Part model, mm, in its own coordinate system. Give positions to 0.01 mm unless a question says otherwise; leave off trailing zeros. Order: outer loops, then holes, each group sorted by start corner. A loop starts at its lowest first (then second) coordinate and runs counter-clockwise, first axis right, second up. Notation, with made-up numbers: M 37.5,36 L 53.5,36 A12 ccw 53.5,53 Z; hole C 16.25,77 d11. An arc over 180 degrees is marked long. Answer as a JSON object with one key per item and string values.
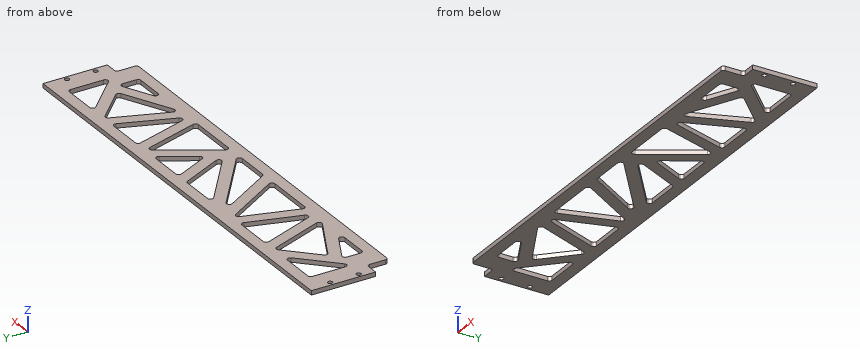
from build123d import *

# Parameters (mm, degrees)
SKETCH_1_W              = 306
SKETCH_1_H              = 60
EXTRUDE_1_DEPTH         = 3
HOLE_WIZARD_3_2_3_2_1_D = 3.2
SKETCH_4_W              = 10
SKETCH_4_H              = 15
CUT_EXTRUDE_1_DEPTH     = 156.94229702
FILLET_1_R              = 2
FILLET_2_R              = 2


with BuildPart() as part:
    # 草图1 → 凸台-拉伸1 (new body)
    with BuildSketch(Plane.XY):
        Rectangle(SKETCH_1_W, SKETCH_1_H)
    extrude(amount=EXTRUDE_1_DEPTH)

    # Ø3.2 (3.2) 直径孔1 (through all)
    with Locations(Plane(origin=(-150, 15, 3), x_dir=(1, 0, 0), z_dir=(0, 0, 1))):
        with Locations((0, 0), (0, -20), (300, 0), (300, -20)):
            Hole(HOLE_WIZARD_3_2_3_2_1_D / 2)

    # 草图4 → 切除-拉伸1 (cut, through all)
    with BuildSketch(Plane.XY.offset(3)):
        Polygon((-138, 22), (-138, -8), (-108, 22), align=None)
        with Locations((-148, -22.5)):
            Rectangle(SKETCH_4_W, SKETCH_4_H)
        Polygon((-128, -7), (-128, -22), (-98, -22), align=None)
        Polygon((-120.494679727, -1.808388226), (-80.11145618, -22), (-96.686291501, 22), align=None)
        Polygon((-88.137500729, 22), (-58.137500729, 22), (-71.562665408, -22), align=None)
        Polygon((-49.773399859, 22), (-63.198564538, -22), (-23.198564538, -22), align=None)
        Polygon((23.198564538, -22), (49.773399859, 22), (63.198564538, -22), align=None)
        Polygon((71.562665408, -22), (88.137500729, 22), (58.137500729, 22), align=None)
        Polygon((96.686291501, 22), (120.494679727, -1.808388226), (80.11145618, -22), align=None)
        Polygon((98, -22), (128, -7), (128, -22), align=None)
        Polygon((108, 22), (138, 22), (138, -8), align=None)
        with Locations((148, -22.5)):
            Rectangle(SKETCH_4_W, SKETCH_4_H)
        Polygon((-40.427482162, 22), (-13.852646841, -22), (16.147353159, -22), align=None)
        Polygon((-27.396416938, 22), (20.1778764, -15), (2.603583062, 22), align=None)
        Polygon((11.460153437, 22), (24.21224704, -4.847592346), (40.427482162, 22), align=None)
    extrude(amount=-CUT_EXTRUDE_1_DEPTH, mode=Mode.SUBTRACT)

    # 圆角1
    fillet_1_edges = [part.edges().sort_by_distance(p)[0] for p in [
        (128, -22, 1.5),
        (98, -22, 1.5),
        (128, -7, 1.5),
        (138, -8, 1.5),
        (108, 22, 1.5),
        (138, 22, 1.5),
        (11.460153437, 22, 1.5),
        (40.427482162, 22, 1.5),
        (24.21224704, -4.847592346, 1.5),
        (-27.396416938, 22, 1.5),
        (2.603583062, 22, 1.5),
        (20.1778764, -15, 1.5),
        (-120.494679727, -1.808388226, 1.5),
        (-96.686291501, 22, 1.5),
        (-80.11145618, -22, 1.5),
        (-71.562665408, -22, 1.5),
        (-88.137500729, 22, 1.5),
        (-58.137500729, 22, 1.5),
        (-138, 22, 1.5),
        (-108, 22, 1.5),
        (-138, -8, 1.5),
        (-128, -7, 1.5),
        (-98, -22, 1.5),
        (-128, -22, 1.5),
        (71.562665408, -22, 1.5),
        (58.137500729, 22, 1.5),
        (88.137500729, 22, 1.5),
        (80.11145618, -22, 1.5),
        (96.686291501, 22, 1.5),
        (120.494679727, -1.808388226, 1.5),
        (63.198564538, -22, 1.5),
        (23.198564538, -22, 1.5),
        (49.773399859, 22, 1.5),
        (-49.773399859, 22, 1.5),
        (-23.198564538, -22, 1.5),
        (-63.198564538, -22, 1.5),
        (-40.427482162, 22, 1.5),
        (16.147353159, -22, 1.5),
        (-13.852646841, -22, 1.5),
    ]]
    fillet(fillet_1_edges, radius=FILLET_1_R)

    # 圆角2
    fillet_2_edges = [part.edges().sort_by_distance(p)[0] for p in [
        (-143, -15, 1.5),
        (-143, -30, 1.5),
        (143, -30, 1.5),
        (143, -15, 1.5),
    ]]
    fillet(fillet_2_edges, radius=FILLET_2_R)


solid = part.part
1. Probe line 1 along Y through (x, z) = (-150, 2.05); line 2 along Y through (x, z) = (50, 0.8); line 3 along Y through (x, z) = (29.5, 2.05). List the from-to ranges inside material, lowest first.
Worked answers:
{"line 1": "y = -15 to -6.6, -3.4 to 13.4, 16.6 to 30", "line 2": "y = -30 to -22, 18.95 to 30", "line 3": "y = -30 to -22, -11.57 to 3.91, 22 to 30"}
2. Cut at B-B on z = 1.05. State how many separate pieces and enclosed holes the cut face has, plus the area to 3 significant figures.
Worked answers:
{"separate pieces": "1", "enclosed holes": "17", "area": "10,700 mm^2"}
3. Cut at A-A on x = -65. Give the cut face in (y, z).
Worked answers:
{"outline": "M -30,0 L -0.49,0 L -0.49,3 L -30,3 Z; M 22,0 L 30,0 L 30,3 L 22,3 Z"}
4. Pin check, flat tips, straight feed: P1, Ø3, axis at x = 150, y = -5, coming from the -Z side; P2, Ø1.5, axis at y = -21, z = 1.5, coming from the -X side. Stop position of each tip, or through.
Worked answers:
{"P1": "passes through", "P2": "stops at x = -143"}
